```python
from build123d import *

# Parameters (mm, degrees)
BOSS_EXTRUDE1_DEPTH = 1.4
BOSS_EXTRUDE2_DEPTH = 0.7
SKETCH3_R           = 0.5
SKETCH3_R_2         = 2.5
BOSS_EXTRUDE3_DEPTH = 0.6
SKETCH4_R           = 2
SKETCH4_R_2         = 0.5
SKETCH4_W           = 2
SKETCH4_H           = 1
BOSS_EXTRUDE4_DEPTH = 1


with BuildPart() as part:
    # Sketch1 → Boss-Extrude1 (new body)
    with BuildSketch(Plane.XY):
        with BuildLine():
            Line((-5.5, 5.809475019), (-5.5, -2.5))
            Line((-5.5, -2.5), (-2.5, -5.5))
            Line((-2.5, -5.5), (2.5, -5.5))
            Line((2.5, -5.5), (5.5, -2.5))
            Line((5.5, -2.5), (5.5, 5.809475019))
            ThreePointArc((5.5, 5.809475019), (0, -8), (-5.5, 5.809475019))
        make_face()
    extrude(amount=BOSS_EXTRUDE1_DEPTH)

    # Sketch2 → Boss-Extrude2 (add)
    with BuildSketch(Plane.XY.offset(1.4)):
        with BuildLine():
            Line((-1, -5.5), (-1, -6.5))
            Line((-1, -6.5), (1, -6.5))
            Line((1, -6.5), (1, -5.5))
            Line((1, -5.5), (2.5, -5.5))
            Line((2.5, -5.5), (5.5, -2.5))
            Line((5.5, -2.5), (5.5, 5.809475019))
            ThreePointArc((5.5, 5.809475019), (0, -8), (-5.5, 5.809475019))
            Line((-5.5, 5.809475019), (-5.5, -2.5))
            Line((-5.5, -2.5), (-2.5, -5.5))
            Line((-2.5, -5.5), (-1, -5.5))
        make_face()
    extrude(amount=BOSS_EXTRUDE2_DEPTH)

    # Sketch3 → Boss-Extrude3 (add)
    # profile 1 of 2: a face of its own
    with BuildSketch(Plane.XY.offset(2.1)):
        Polygon((2.5, -5.5), (5.5, -2.5), (5.5, 6.5), (-5.5, 6.5), (-5.5, -2.5), (-2.5, -5.5), align=None)
        with Locations((4.250000001, 5.5)):
            Circle(SKETCH3_R, mode=Mode.SUBTRACT)
        Circle(SKETCH3_R_2, mode=Mode.SUBTRACT)
        with Locations((-4.249999999, 5.5)):
            Circle(SKETCH3_R, mode=Mode.SUBTRACT)
    # profile 2 of 2: a face of its own
    with BuildSketch(Plane.XY.offset(2.1)):
        with BuildLine():
            Line((-1, -6.5), (-1, -5.5))
            Line((-1, -5.5), (-2.5, -5.5))
            Line((-2.5, -5.5), (-5.5, -2.5))
            Line((-5.5, -2.5), (-5.5, 5.809475019))
            ThreePointArc((-5.5, 5.809475019), (0, -8), (5.5, 5.809475019))
            Line((5.5, 5.809475019), (5.5, -2.5))
            Line((5.5, -2.5), (2.5, -5.5))
            Line((2.5, -5.5), (1, -5.5))
            Line((1, -5.5), (1, -6.5))
            Line((1, -6.5), (-1, -6.5))
        make_face()
    extrude(amount=BOSS_EXTRUDE3_DEPTH)

    # Sketch4 → Boss-Extrude4 (add)
    with BuildSketch(Plane.XY.offset(2.7)):
        with BuildLine():
            Line((-5.5, 5.809475019), (-5.5, 6.5))
            Line((-5.5, 6.5), (5.5, 6.5))
            Line((5.5, 6.5), (5.5, 5.809475019))
            ThreePointArc((5.5, 5.809475019), (0, -8), (-5.5, 5.809475019))
        make_face()
        Circle(SKETCH4_R, mode=Mode.SUBTRACT)
        with Locations((-4.249999999, 5.5)):
            Circle(SKETCH4_R_2, mode=Mode.SUBTRACT)
        with Locations((4.250000001, 5.5)):
            Circle(SKETCH4_R_2, mode=Mode.SUBTRACT)
        with Locations((0, -6)):
            Rectangle(SKETCH4_W, SKETCH4_H, mode=Mode.SUBTRACT)
    extrude(amount=BOSS_EXTRUDE4_DEPTH)


solid = part.part
```
Design review of the part built by this model. Coordinates are the model's own, in mm. A direction names the side the tool comes from. Round coordinates to 2 decimals unless told otherwise and drop trailing zeros. Write each loop counter-clockwise with the first axis right and the second up, starting at its lowest first coordinate (ties: lowest second). Pieces come first, ordered by that corner, then holes.
Item 1: We need section B-B on y = 0. Write out the cut boundary in (x, z), and give its area (3 significant figures).
Item 2: Clearance check with flat-ended pins moving along their axes: pin 1 Ø1.7 at (y, z) = (3.5, 0.5) entering from -X; pin 2 Ø1.5 at (x, z) = (3, 3) entering from -Y; pin 3 Ø1 at (y, z) = (1.5, 1) entering from +X. State where each tip first meets the part, or that it passes through.
Item 3: For probe 1 along Y at (x, z) = (0, 2.4); probe 2 along Z at (x, y) = (-1.25, -4); probe 3 along Y at (x, z) = (0.5, 2.8), list the stretches that pass through material, from the lowest coordinate up.
Item 4: We need section C-C on z = 2.5. Write out the cut boundary in (x, y).
Item 5: We need section D-D on x = 4.25. Write out the cut boundary in (y, z), and give its area (3 significant figures).
Item 6: For faces 3 (the flat face through (0, -6, 0)), 4 (the flat face through (0, 3, 2.1)), 5 (the flat face through (0, -6, 1.4)), 6 (the cylindrical face through (-0.54, -2.44, 2.4)), list the 3-axis set-ups (+Z, -Z, +X, -X, +Y, -Y) from which the entire face can be reached by the end or side of a thin tool; tool diameter is ignored.
Item 7: The part is to be moulded in two halves that separate along X. For faces 1 (the flat face through (0.1, -2.3, 3.7)), 2 (the flat face through (1, 2, 2.7)), say which applies: +X half, -X half, draft (parallel to the pull), parting line (faces both ways), or undercut.
Item 8: We need section A-A on x = 0. Write out the cut boundary in (y, z).
Returned:
1. outline: (-8, 0) - (-5.5, 0) - (-5.5, 2.1) - (-2.5, 2.1) - (-2.5, 2.7) - (-2, 2.7) - (-2, 3.7) - (-8, 3.7) - close; (2, 2.7) - (2.5, 2.7) - (2.5, 2.1) - (5.5, 2.1) - (5.5, 0) - (8, 0) - (8, 3.7) - (2, 3.7) - close
1. area: 29.1 mm2
2. pin 1: stops at x = -7.55
2. pin 2: stops at y = -7.68
2. pin 3: stops at x = 7.94
3. probe 1: y = -8 to -6.5, -5.5 to -2.5, 2.5 to 6.5
3. probe 2: z = 2.1 to 3.7
3. probe 3: y = -7.98 to -6.5, -5.5 to -1.94, 1.94 to 6.5
4. outline: (-5.5, 5.81) arc R8 ccw (long way) to (5.5, 5.81) - (5.5, 6.5) - (-5.5, 6.5) - close; hole circle Ø1 at (-4.25, 5.5); hole circle Ø5 at (0, 0); hole (-1, -6.5) - (1, -6.5) - (1, -5.5) - (-1, -5.5) - close; hole circle Ø1 at (4.25, 5.5)
5. outline: (-6.78, 0) - (-3.75, 0) - (-3.75, 2.1) - (5, 2.1) - (5, 3.7) - (-6.78, 3.7) - close; (6, 2.1) - (6.5, 2.1) - (6.5, 3.7) - (6, 3.7) - close
5. area: 26.0 mm2
6. face 3: -Z, +X, -X, +Y, -Y
6. face 4: -Z, +Y
6. face 5: +Z, +Y
6. face 6: -Z
7. face 1: draft
7. face 2: undercut
8. outline: (-8, 0) - (-5.5, 0) - (-5.5, 1.4) - (-6.5, 1.4) - (-6.5, 3.7) - (-8, 3.7) - close; (-5.5, 2.1) - (-2.5, 2.1) - (-2.5, 2.7) - (-2, 2.7) - (-2, 3.7) - (-5.5, 3.7) - close; (2, 2.7) - (2.5, 2.7) - (2.5, 2.1) - (6.5, 2.1) - (6.5, 3.7) - (2, 3.7) - close
